Source: CAD feature listing. Evaluate the final solid. Frame: model axes, mm. Face numbers are marked on the shaded views. A direction names the side the tool comes from. Give positions to 0.01 mm unless a question says otherwise; leave off trailing zeros. Order: outer loops, then holes, each group sorted by start corner. A loop starts at its lowest first (then second) coordinate and runs counter-clockwise, first axis right, second up.
1) Access query for the marked faces 1, 2 and 3. Directions: +Z, -Z, +X, -X, +Y, -Y. A direction counts if a zero-diameter tool reaches every point of the face in a straight line with its end or side. Return the directions, or none.
2) First-contact query: P1, Ø1.2, axis at x = -33.5, z = 2, coming from the -Y side; P2, Ø1.1, axis at y = 3, z = 4.5, coming from the -X side; P3, Ø3, axis at y = 5, z = 4.5, coming from the -X side; P4, Ø1, axis at x = -25, y = 6, coming from the -Z side. Flat tips, straight axial feed; report the tip coordinate or a pass-through.
3) Section A-A, the plane x = -33.5. Return loops of the section in (y, z).
4) Draft query along X for the marked faces 4, 5 and 6. Return one class per face: released by +X, released by -X, zero draft, split by the parting line, or undercut.
5) Section C-C, the plane z = 2. Return loops of the section in (x, y).
6) Section B-B, the plane y = 8.5. Return loops of the section in (x, z).
7) Section D-D, the plane y = 12.5. Return loops of the section in (x, z).
8) Material intervals for line 1 (Z direction, x = -2.5, y = 9.5); line 2 (X direction, y = 13.75, z = 5); line 3 (X direction, y = 9.5, z = 5), sorted ascending.
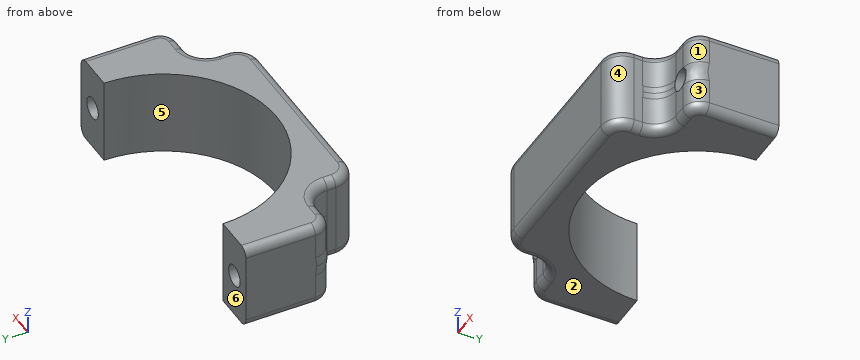
```python
from build123d import *

# Parameters (mm, degrees)
PAD_DEPTH    = 10
SKETCH_R     = 1.25
POCKET_DEPTH = 16.001
FILLET_R     = 2.5
FILLET001_R  = 2.5
FILLET002_R  = 2.5
FILLET003_R  = 2.5
FILLET004_R  = 2
FILLET005_R  = 2
FILLET006_R  = 1
FILLET007_R  = 1


with BuildPart() as part:
    # Sketch001 → Pad (new body)
    with BuildSketch(Plane.XY):
        with BuildLine():
            Line((-36, 16), (-31, 16))
            ThreePointArc((-31, 16), (-18, 3), (-5, 16))
            Line((0, 16), (-5, 16))
            Line((0, 6), (0, 16))
            Line((-6, 6), (0, 6))
            Line((-6, 0), (-6, 6))
            Line((-30, 0), (-6, 0))
            Line((-30, 6), (-30, 0))
            Line((-36, 6), (-30, 6))
            Line((-36, 6), (-36, 16))
        make_face()
    extrude(amount=PAD_DEPTH)

    # Sketch (on Face4 of Pad) → Pocket (cut, through all)
    with BuildSketch(Plane(origin=(0, 16, 0), x_dir=(-1, 0, 0), z_dir=(0, 1, 0))):
        with Locations((2.5, 5)):
            Circle(SKETCH_R)
        with Locations((33.5, 5)):
            Circle(SKETCH_R)
    extrude(amount=-POCKET_DEPTH, mode=Mode.SUBTRACT)

    # Fillet
    fillet_edges = [part.edges().sort_by_distance(p)[0] for p in [
        (-6, 6, 5),
    ]]
    fillet(fillet_edges, radius=FILLET_R)

    # Fillet001
    fillet001_edges = [part.edges().sort_by_distance(p)[0] for p in [
        (-6, 0, 5),
    ]]
    fillet(fillet001_edges, radius=FILLET001_R)

    # Fillet002
    fillet002_edges = [part.edges().sort_by_distance(p)[0] for p in [
        (-30, 6, 5),
    ]]
    fillet(fillet002_edges, radius=FILLET002_R)

    # Fillet003
    fillet003_edges = [part.edges().sort_by_distance(p)[0] for p in [
        (-30, 0, 5),
    ]]
    fillet(fillet003_edges, radius=FILLET003_R)

    # Fillet004
    fillet004_edges = [part.edges().sort_by_distance(p)[0] for p in [
        (-36, 6, 5),
    ]]
    fillet(fillet004_edges, radius=FILLET004_R)

    # Fillet005
    fillet005_edges = [part.edges().sort_by_distance(p)[0] for p in [
        (0, 6, 5),
    ]]
    fillet(fillet005_edges, radius=FILLET005_R)

    # Fillet006
    fillet006_edges = [part.edges().sort_by_distance(p)[0] for p in [
        (-35.414214, 6.585786, 10),
    ]]
    fillet(fillet006_edges, radius=FILLET006_R)

    # Fillet007
    fillet007_edges = [part.edges().sort_by_distance(p)[0] for p in [
        (-30.732233, 5.267767, 0),
    ]]
    fillet(fillet007_edges, radius=FILLET007_R)


solid = part.part
```
From the geometry:
1. face 1: +Z, +X, -Y
1. face 2: -Z, +X, -X, +Y, -Y
1. face 3: -Z, +X, -Y
2. P1: stops at y = 6
2. P2: stops at x = -30
2. P3: stops at x = -35.45
2. P4: passes through
3. outline: (6, 1) arc R1 ccw to (7, 0) - (16, 0) - (16, 3.75) - (6, 3.75) - close; (6, 6.25) - (16, 6.25) - (16, 10) - (7, 10) arc R1 ccw to (6, 9) - close
4. face 4: released by +X
4. face 5: undercut
4. face 6: zero draft
5. outline: (-36, 8) arc R2 ccw to (-34, 6) - (-32.5, 6) arc R2.5 cw to (-30, 3.5) - (-30, 2.5) arc R2.5 ccw to (-27.5, 0) - (-8.5, 0) arc R2.5 ccw to (-6, 2.5) - (-6, 3.5) arc R2.5 cw to (-3.5, 6) - (-2, 6) arc R2 ccw to (0, 8) - (0, 16) - (-5, 16) arc R13 cw to (-31, 16) - (-36, 16) - close
6. outline: (-36, 1) arc R1 ccw to (-35, 0) - (-28.62, 0) - (-28.62, 10) - (-35, 10) arc R1 ccw to (-36, 9) - close; (-7.38, 0) - (-1, 0) arc R1 ccw to (0, 1) - (0, 9) arc R1 ccw to (-1, 10) - (-7.38, 10) - close; hole circle Ø2.5 at (-33.5, 5); hole circle Ø2.5 at (-2.5, 5)
7. outline: (-36, 1) arc R1 ccw to (-35, 0) - (-30.52, 0) - (-30.52, 10) - (-35, 10) arc R1 ccw to (-36, 9) - close; (-5.48, 0) - (-1, 0) arc R1 ccw to (0, 1) - (0, 9) arc R1 ccw to (-1, 10) - (-5.48, 10) - close; hole circle Ø2.5 at (-33.5, 5); hole circle Ø2.5 at (-2.5, 5)
8. line 1: z = 0 to 3.75, 6.25 to 10
8. line 2: x = -36 to -34.75, -32.25 to -30.8, -5.2 to -3.75, -1.25 to 0
8. line 3: x = -36 to -34.75, -32.25 to -29.26, -6.74 to -3.75, -1.25 to 0
